from build123d import *

# Parameters (mm, degrees)
SKETCH1_R           = 1
BOSS_EXTRUDE1_DEPTH = 4
SKETCH2_R           = 1
CUT_EXTRUDE1_DEPTH  = 2
BOSS_EXTRUDE2_DEPTH = 2
BOSS_EXTRUDE3_REACH = 89.691


with BuildPart() as part:
    # Sketch1 → Boss-Extrude1 (new body)
    with BuildSketch(Plane.XY):
        with BuildLine():
            Line((-56.056622595, 63.083032854), (-4.020390364, 33.212804613))
            ThreePointArc((-4.020390364, 33.212804613), (-3.096806864, 29.800035426), (-6.509576051, 28.876451927))
            Line((-6.509576051, 28.876451927), (-58.545808282, 58.746680168))
            ThreePointArc((-58.545808282, 58.746680168), (-59.469391781, 62.159449355), (-56.056622595, 63.083032854))
        make_face()
        with Locations((-57.301215438, 60.914856511)):
            Circle(SKETCH1_R, mode=Mode.SUBTRACT)
        with Locations((-5.264983207, 31.04462827)):
            Circle(SKETCH1_R, mode=Mode.SUBTRACT)
    extrude(amount=BOSS_EXTRUDE1_DEPTH)

    # Sketch2 → Cut-Extrude1 (cut)
    with BuildSketch(Plane(origin=(13.343522454, 23.245441166, 0), x_dir=(0.8672705371832455, -0.49783713735908147, 0), z_dir=(0.49783713735908147, 0.8672705371832455, 0))):
        with Locations(Location((-48.403705156, -2, 0), (0, 0, 180))):
            Circle(SKETCH2_R)
    extrude(amount=-CUT_EXTRUDE1_DEPTH, mode=Mode.SUBTRACT)

    # Sketch4 → Boss-Extrude2 (add)
    with BuildSketch(Plane(origin=(10.854336767, 18.90908848, 0), x_dir=(0.8672705371832455, -0.49783713735908136, 0), z_dir=(-0.49783713735908136, -0.8672705371832455, 0))):
        with BuildLine():
            Line((-73.918626185, 6.8), (-34.010435963, 6.8))
            ThreePointArc((-34.010435963, 6.8), (-33.372509372, 4.895560129), (-31.574784807, 4))
            Line((-31.574784807, 4), (-31.574784807, 0))
            ThreePointArc((-31.574784807, 0), (-33.372509372, -0.895560129), (-34.010435963, -2.8))
            Line((-34.010435963, -2.8), (-73.918626185, -2.8))
            ThreePointArc((-73.918626185, -2.8), (-74.749293349, -0.809525322), (-76.748459708, 0))
            Line((-76.748459708, 0), (-75.579913588, 4))
            ThreePointArc((-75.579913588, 4), (-74.306304145, 5.137180927), (-73.918626185, 6.8))
        make_face()
    extrude(amount=-BOSS_EXTRUDE2_DEPTH)

    # Boss-Extrude3: up to this face of the body (flat: up to its plane)
    boss_extrude3_end = Plane(part.part.faces().sort_by_distance((-35.449673949, 46.641906686, 6.8))[0])
    # Sketch5 → Boss-Extrude3 (add, up to the picked face)
    with BuildSketch(Plane(origin=(0, 0, -2.8), x_dir=(-1, 0, 0), z_dir=(0, 0, -1)), mode=Mode.PRIVATE) as boss_extrude3_sk1:
        Polygon((52.899098519, 55.505313486), (51.164557445, 54.509639211), (52.529665119, 54.140205811), align=None)
    boss_extrude3_tool1 = split(extrude(boss_extrude3_sk1.sketch, amount=-BOSS_EXTRUDE3_REACH, mode=Mode.PRIVATE), bisect_by=boss_extrude3_end, keep=Keep.BOTH, mode=Mode.PRIVATE)
    # Sketch5 → Boss-Extrude3 (add, up to the picked face)
    with BuildSketch(Plane(origin=(0, 0, -2.8), x_dir=(-1, 0, 0), z_dir=(0, 0, -1)), mode=Mode.PRIVATE) as boss_extrude3_sk2:
        Polygon((18.6419123, 35.84074656), (20.007019975, 35.47131316), (20.376453374, 36.836420835), align=None)
    boss_extrude3_tool2 = split(extrude(boss_extrude3_sk2.sketch, amount=-BOSS_EXTRUDE3_REACH, mode=Mode.PRIVATE), bisect_by=boss_extrude3_end, keep=Keep.BOTH, mode=Mode.PRIVATE)
    # Sketch5 → Boss-Extrude3 (add, up to the picked face)
    with BuildSketch(Plane(origin=(0, 0, -2.8), x_dir=(-1, 0, 0), z_dir=(0, 0, -1)), mode=Mode.PRIVATE) as boss_extrude3_sk3:
        Polygon((20.810088643, 37.085339404), (22.175196318, 36.715906004), (22.544629717, 38.081013678), align=None)
    boss_extrude3_tool3 = split(extrude(boss_extrude3_sk3.sketch, amount=-BOSS_EXTRUDE3_REACH, mode=Mode.PRIVATE), bisect_by=boss_extrude3_end, keep=Keep.BOTH, mode=Mode.PRIVATE)
    # Sketch5 → Boss-Extrude3 (add, up to the picked face)
    with BuildSketch(Plane(origin=(0, 0, -2.8), x_dir=(-1, 0, 0), z_dir=(0, 0, -1)), mode=Mode.PRIVATE) as boss_extrude3_sk4:
        Polygon((22.978264986, 38.329932247), (24.343372661, 37.960498847), (24.71280606, 39.325606522), align=None)
    boss_extrude3_tool4 = split(extrude(boss_extrude3_sk4.sketch, amount=-BOSS_EXTRUDE3_REACH, mode=Mode.PRIVATE), bisect_by=boss_extrude3_end, keep=Keep.BOTH, mode=Mode.PRIVATE)
    # Sketch5 → Boss-Extrude3 (add, up to the picked face)
    with BuildSketch(Plane(origin=(0, 0, -2.8), x_dir=(-1, 0, 0), z_dir=(0, 0, -1)), mode=Mode.PRIVATE) as boss_extrude3_sk5:
        Polygon((25.146441329, 39.57452509), (26.511549004, 39.205091691), (26.880982403, 40.570199365), align=None)
    boss_extrude3_tool5 = split(extrude(boss_extrude3_sk5.sketch, amount=-BOSS_EXTRUDE3_REACH, mode=Mode.PRIVATE), bisect_by=boss_extrude3_end, keep=Keep.BOTH, mode=Mode.PRIVATE)
    # Sketch5 → Boss-Extrude3 (add, up to the picked face)
    with BuildSketch(Plane(origin=(0, 0, -2.8), x_dir=(-1, 0, 0), z_dir=(0, 0, -1)), mode=Mode.PRIVATE) as boss_extrude3_sk6:
        Polygon((27.314617672, 40.819117934), (28.679725347, 40.449684534), (29.049158746, 41.814792208), align=None)
    boss_extrude3_tool6 = split(extrude(boss_extrude3_sk6.sketch, amount=-BOSS_EXTRUDE3_REACH, mode=Mode.PRIVATE), bisect_by=boss_extrude3_end, keep=Keep.BOTH, mode=Mode.PRIVATE)
    # Sketch5 → Boss-Extrude3 (add, up to the picked face)
    with BuildSketch(Plane(origin=(0, 0, -2.8), x_dir=(-1, 0, 0), z_dir=(0, 0, -1)), mode=Mode.PRIVATE) as boss_extrude3_sk7:
        Polygon((29.482794015, 42.063710777), (30.847901689, 41.694277377), (31.217335089, 43.059385052), align=None)
    boss_extrude3_tool7 = split(extrude(boss_extrude3_sk7.sketch, amount=-BOSS_EXTRUDE3_REACH, mode=Mode.PRIVATE), bisect_by=boss_extrude3_end, keep=Keep.BOTH, mode=Mode.PRIVATE)
    # Sketch5 → Boss-Extrude3 (add, up to the picked face)
    with BuildSketch(Plane(origin=(0, 0, -2.8), x_dir=(-1, 0, 0), z_dir=(0, 0, -1)), mode=Mode.PRIVATE) as boss_extrude3_sk8:
        Polygon((31.650970358, 43.308303621), (33.016078032, 42.938870221), (33.385511432, 44.303977895), align=None)
    boss_extrude3_tool8 = split(extrude(boss_extrude3_sk8.sketch, amount=-BOSS_EXTRUDE3_REACH, mode=Mode.PRIVATE), bisect_by=boss_extrude3_end, keep=Keep.BOTH, mode=Mode.PRIVATE)
    # Sketch5 → Boss-Extrude3 (add, up to the picked face)
    with BuildSketch(Plane(origin=(0, 0, -2.8), x_dir=(-1, 0, 0), z_dir=(0, 0, -1)), mode=Mode.PRIVATE) as boss_extrude3_sk9:
        Polygon((33.819146701, 44.552896464), (35.184254375, 44.183463064), (35.553687775, 45.548570739), align=None)
    boss_extrude3_tool9 = split(extrude(boss_extrude3_sk9.sketch, amount=-BOSS_EXTRUDE3_REACH, mode=Mode.PRIVATE), bisect_by=boss_extrude3_end, keep=Keep.BOTH, mode=Mode.PRIVATE)
    # Sketch5 → Boss-Extrude3 (add, up to the picked face)
    with BuildSketch(Plane(origin=(0, 0, -2.8), x_dir=(-1, 0, 0), z_dir=(0, 0, -1)), mode=Mode.PRIVATE) as boss_extrude3_sk10:
        Polygon((35.987323044, 45.797489307), (37.352430718, 45.428055908), (37.721864118, 46.793163582), align=None)
    boss_extrude3_tool10 = split(extrude(boss_extrude3_sk10.sketch, amount=-BOSS_EXTRUDE3_REACH, mode=Mode.PRIVATE), bisect_by=boss_extrude3_end, keep=Keep.BOTH, mode=Mode.PRIVATE)
    # Sketch5 → Boss-Extrude3 (add, up to the picked face)
    with BuildSketch(Plane(origin=(0, 0, -2.8), x_dir=(-1, 0, 0), z_dir=(0, 0, -1)), mode=Mode.PRIVATE) as boss_extrude3_sk11:
        Polygon((38.155499387, 47.042082151), (39.520607061, 46.672648751), (39.890040461, 48.037756425), align=None)
    boss_extrude3_tool11 = split(extrude(boss_extrude3_sk11.sketch, amount=-BOSS_EXTRUDE3_REACH, mode=Mode.PRIVATE), bisect_by=boss_extrude3_end, keep=Keep.BOTH, mode=Mode.PRIVATE)
    # Sketch5 → Boss-Extrude3 (add, up to the picked face)
    with BuildSketch(Plane(origin=(0, 0, -2.8), x_dir=(-1, 0, 0), z_dir=(0, 0, -1)), mode=Mode.PRIVATE) as boss_extrude3_sk12:
        Polygon((40.32367573, 48.286674994), (41.688783404, 47.917241594), (42.058216804, 49.282349269), align=None)
    boss_extrude3_tool12 = split(extrude(boss_extrude3_sk12.sketch, amount=-BOSS_EXTRUDE3_REACH, mode=Mode.PRIVATE), bisect_by=boss_extrude3_end, keep=Keep.BOTH, mode=Mode.PRIVATE)
    # Sketch5 → Boss-Extrude3 (add, up to the picked face)
    with BuildSketch(Plane(origin=(0, 0, -2.8), x_dir=(-1, 0, 0), z_dir=(0, 0, -1)), mode=Mode.PRIVATE) as boss_extrude3_sk13:
        Polygon((42.491852073, 49.531267838), (43.856959747, 49.161834438), (44.226393147, 50.526942112), align=None)
    boss_extrude3_tool13 = split(extrude(boss_extrude3_sk13.sketch, amount=-BOSS_EXTRUDE3_REACH, mode=Mode.PRIVATE), bisect_by=boss_extrude3_end, keep=Keep.BOTH, mode=Mode.PRIVATE)
    # Sketch5 → Boss-Extrude3 (add, up to the picked face)
    with BuildSketch(Plane(origin=(0, 0, -2.8), x_dir=(-1, 0, 0), z_dir=(0, 0, -1)), mode=Mode.PRIVATE) as boss_extrude3_sk14:
        Polygon((44.660028416, 50.775860681), (46.02513609, 50.406427281), (46.39456949, 51.771534956), align=None)
    boss_extrude3_tool14 = split(extrude(boss_extrude3_sk14.sketch, amount=-BOSS_EXTRUDE3_REACH, mode=Mode.PRIVATE), bisect_by=boss_extrude3_end, keep=Keep.BOTH, mode=Mode.PRIVATE)
    # Sketch5 → Boss-Extrude3 (add, up to the picked face)
    with BuildSketch(Plane(origin=(0, 0, -2.8), x_dir=(-1, 0, 0), z_dir=(0, 0, -1)), mode=Mode.PRIVATE) as boss_extrude3_sk15:
        Polygon((46.828204759, 52.020453524), (48.193312433, 51.651020125), (48.562745833, 53.016127799), align=None)
    boss_extrude3_tool15 = split(extrude(boss_extrude3_sk15.sketch, amount=-BOSS_EXTRUDE3_REACH, mode=Mode.PRIVATE), bisect_by=boss_extrude3_end, keep=Keep.BOTH, mode=Mode.PRIVATE)
    # Sketch5 → Boss-Extrude3 (add, up to the picked face)
    with BuildSketch(Plane(origin=(0, 0, -2.8), x_dir=(-1, 0, 0), z_dir=(0, 0, -1)), mode=Mode.PRIVATE) as boss_extrude3_sk16:
        Polygon((48.996381102, 53.265046368), (50.361488776, 52.895612968), (50.730922176, 54.260720642), align=None)
    boss_extrude3_tool16 = split(extrude(boss_extrude3_sk16.sketch, amount=-BOSS_EXTRUDE3_REACH, mode=Mode.PRIVATE), bisect_by=boss_extrude3_end, keep=Keep.BOTH, mode=Mode.PRIVATE)
    add(boss_extrude3_tool1.solids().sort_by(Axis((-52.197774, 54.718386, -2.8), (0, 0, 1)))[0])
    add(boss_extrude3_tool2.solids().sort_by(Axis((-19.675129, 36.049494, -2.8), (0, 0, 1)))[0])
    add(boss_extrude3_tool3.solids().sort_by(Axis((-21.843305, 37.294086, -2.8), (0, 0, 1)))[0])
    add(boss_extrude3_tool4.solids().sort_by(Axis((-24.011481, 38.538679, -2.8), (0, 0, 1)))[0])
    add(boss_extrude3_tool5.solids().sort_by(Axis((-26.179658, 39.783272, -2.8), (0, 0, 1)))[0])
    add(boss_extrude3_tool6.solids().sort_by(Axis((-28.347834, 41.027865, -2.8), (0, 0, 1)))[0])
    add(boss_extrude3_tool7.solids().sort_by(Axis((-30.51601, 42.272458, -2.8), (0, 0, 1)))[0])
    add(boss_extrude3_tool8.solids().sort_by(Axis((-32.684187, 43.517051, -2.8), (0, 0, 1)))[0])
    add(boss_extrude3_tool9.solids().sort_by(Axis((-34.852363, 44.761643, -2.8), (0, 0, 1)))[0])
    add(boss_extrude3_tool10.solids().sort_by(Axis((-37.020539, 46.006236, -2.8), (0, 0, 1)))[0])
    add(boss_extrude3_tool11.solids().sort_by(Axis((-39.188716, 47.250829, -2.8), (0, 0, 1)))[0])
    add(boss_extrude3_tool12.solids().sort_by(Axis((-41.356892, 48.495422, -2.8), (0, 0, 1)))[0])
    add(boss_extrude3_tool13.solids().sort_by(Axis((-43.525068, 49.740015, -2.8), (0, 0, 1)))[0])
    add(boss_extrude3_tool14.solids().sort_by(Axis((-45.693245, 50.984608, -2.8), (0, 0, 1)))[0])
    add(boss_extrude3_tool15.solids().sort_by(Axis((-47.861421, 52.2292, -2.8), (0, 0, 1)))[0])
    add(boss_extrude3_tool16.solids().sort_by(Axis((-50.029597, 53.473793, -2.8), (0, 0, 1)))[0])


solid = part.part
Check sheet for the modelled part. Datum: model origin and axes. Units: mm. A direction names the side the tool comes from. Coordinates: 2 decimals unless noted, no trailing zeros. Write each loop counter-clockwise with the first axis right and the second up, starting at its lowest first coordinate (ties: lowest second). Pieces come first, ordered by that corner, then holes.
Item 1: Cross-section at A-A on y = 34. Record the boundary of the cut face in (x, z).
Numbers:
outline: (-15.44, 0) - (-5.39, 0) - (-5.39, 4) - (-15.44, 4) - close
Item 2: Depth check by flat-ended pin: pin 1 Ø6 at (x, y) = (-9, 34.5) entering from -Z; pin 2 Ø1.5 at (x, z) = (-10, 0.5) entering from +Y; pin 3 Ø10.5 at (x, y) = (-27, 37.5) entering from -Z; pin 4 Ø3 at (y, z) = (53, 5.5) entering from -X. Enter the tip coordinate at first touch or a pass-through.
Numbers:
pin 1: stops at z = 0
pin 2: stops at y = 37.08
pin 3: stops at z = -2.8
pin 4: stops at x = -52.63
Item 3: Mould release check, pull along Z, two halves, no side actions. Record for faces 3 (the face through (-29.62, 45.6, 2.01)), 4 (the face through (-40.997, 48.105, 1.933)): released by +Z, released by -Z, zero draft, split by the parting line, or undercut.
Numbers:
face 3: undercut
face 4: zero draft
Item 4: Access from +Z, -Z, +X, -X, +Y, -Y to the whole of each face (thin tool, end or side, straight path). Record for faces 1 (the face through (-49.669, 53.083, 1.933)), 2 (the face through (-34.349, 47.163, 5.42)).
Numbers:
face 1: +Z, -Z, -Y
face 2: +Z, +X, +Y
Item 5: Scan lines: probe 1 along Y at (x, z) = (-30, 2.75); probe 2 along Z at (x, y) = (-53, 60); probe 3 along X at (y, z) = (48.5, 5). Record each from-to range of solid material in increasing order.
Numbers:
probe 1: y = 41.92 to 45.82, 46.29 to 48.13
probe 2: z = 0 to 4
probe 3: x = -41.85 to -36.68
